For this review, take the finished solid that the model builds, in its own axes (mm). Coordinates: 2 decimals unless noted, no trailing zeros. Return JSON: item names as keys, results as strings. Group by question number.
Item 1: Insertion check: pin 1 (4 mm diameter, centred on x = -28.89, y = 10.06, fed in from -Z). The pin has a flat end and moves straight along its axis. Give the tip position at first contact, or say it passes through.
Item 2: Take a section at A-A (z = 2). Count the separate pieces of the cut face and the enclosed holes in it, then the cut area to 3 significant figures.
Item 3: For line 1 along X through (y, z) = (10, 3.9); line 2 along X through (y, z) = (44.5, 3.25); line 3 along Y through (x, z) = (-28.5, 0.8), list the stretches that pass through material, from the lowest coordinate up.
```python
from build123d import *

# Parameters (mm, degrees)
SKETCH1_W               = 40
SKETCH1_H               = 64
BOSS_EXTRUDE1_DEPTH     = 6
SKETCH2_R               = 1.5
CUT_EXTRUDE1_DEPTH      = 1
CUT_EXTRUDE1_DEPTH_BACK = 7


with BuildPart() as part:
    # Sketch1 → Boss-Extrude1 (new body)
    with BuildSketch(Plane.XY):
        with Locations((-12.888888889, 35.555555556)):
            Rectangle(SKETCH1_W, SKETCH1_H)
    extrude(amount=BOSS_EXTRUDE1_DEPTH)

    # Sketch2 → Cut-Extrude1 (cut, two sides)
    with BuildSketch(Plane.XY.offset(6)) as cut_extrude1_sk:
        with Locations((-28.888888889, 10.055555556)):
            Circle(SKETCH2_R)
        with Locations((-28.888888889, 27.055555556)):
            Circle(SKETCH2_R)
        with Locations((-28.888888889, 44.055555556)):
            Circle(SKETCH2_R)
        with Locations((-28.888888889, 61.055555556)):
            Circle(SKETCH2_R)
        with Locations((3.111111111, 10.055555556)):
            Circle(SKETCH2_R)
        with Locations((3.111111111, 27.055555556)):
            Circle(SKETCH2_R)
        with Locations((3.111111111, 44.055555556)):
            Circle(SKETCH2_R)
        with Locations((3.111111111, 61.055555556)):
            Circle(SKETCH2_R)
    extrude(amount=CUT_EXTRUDE1_DEPTH, mode=Mode.SUBTRACT)
    extrude(cut_extrude1_sk.sketch, amount=-CUT_EXTRUDE1_DEPTH_BACK, mode=Mode.SUBTRACT)


solid = part.part
```
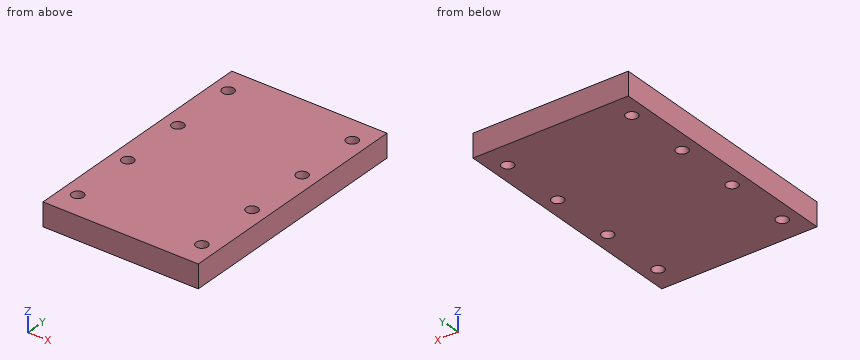
Findings below:
{
 "1": {"pin 1": "stops at z = 0"},
 "2": {"separate pieces": "1", "enclosed holes": "8", "area": "2,500 mm2"},
 "3": {"line 1": "x = -32.89 to -30.39, -27.39 to 1.61, 4.61 to 7.11", "line 2": "x = -32.89 to -30.32, -27.46 to 1.68, 4.54 to 7.11", "line 3": "y = 3.56 to 8.61, 11.5 to 25.61, 28.5 to 42.61, 45.5 to 59.61, 62.5 to 67.56"}
}
